The listing builds one solid part. Answer for the finished solid, in the listing's coordinates (mm). A direction names the side the tool comes from. Give positions to 0.01 mm unless a question says otherwise; leave off trailing zeros. Loops run counter-clockwise (first coordinate to the right, second up) from the corner with the lowest first, then second, coordinate; pieces in that order, holes last.
Item 1: Section A-A, the plane y = -91 is taken. Give the vertices of the cut face in (x, z), and give its area (3 significant figures).
Item 2: Section B-B, the plane x = 27 is taken. Give the vertices of the cut face in (y, z), and give its area (3 significant figures).
Item 3: Section C-C, the plane z = 31 is taken. Give the vertices of the cut face in (x, y).
Item 4: Each of these flat-tipped pins is pushed along its axis until it touches: pin 1 Ø20 at (x, z) = (15, 16) entering from +Y; pin 2 Ø2.5 at (y, z) = (-1.5, 0.5) entering from +X; pin 3 Ø1.5 at (x, y) = (33.5, -141) entering from +Z. Where does it stop, or does it pass through?
Item 5: A tool of negligible diameter and unlimited length cuts with its end or side. For faces 1 (the face through (35.5, -99, 0)), 2 (the face through (0, -32, 1.5)), 3 (the face through (-45.5, -95, 1)), from which of +Z, -Z, +X, -X, +Y, -Y can it reach the whole face along a straight path? Write none if from no direction.
Item 6: Consider line 1 along Y through (x, z) = (-38.5, 16); line 2 along Z through (x, y) = (-40, -45.5). Determine where each line is inside the solid, lowest interval first.
Autodesk Inventor part; units mm, degrees
ref_plane "YZ Plane" through (0, 0, 0) normal (1, 0, 0) x (0, 1, 0)
ref_plane "XZ Plane" through (0, 0, 0) normal (0, 1, 0) x (-1, 0, 0)
ref_plane "XY Plane" through (0, 0, 0) normal (0, 0, 1) x (1, 0, 0)
sketch "Skizze1" plane through (0, 0, 0) normal (0, 0, 1) x (1, 0, 0)
  line L0 (-45.5, 35.5) -> (45.5, 35.5)
  line L1 (45.5, 35.5) -> (45.5, -35.5)
  line L2 (45.5, -35.5) -> (-45.5, -35.5)
  line L3 (-45.5, -35.5) -> (-45.5, 35.5)
  line L4 (-45.5, 35.5) -> (45.5, -35.5) construction
  line L5 (45.5, 35.5) -> (-45.5, -35.5) construction
  line L6 (-34.8, 25.15) -> (45.5, 25.15)
  line L7 (-34.8, -25.15) -> (45.5, -25.15)
  line L8 (0, 0) -> (46.8412, 0)
  line L9 (-34.8, 25.15) -> (-34.8, -25.15)
  line L10 (-31.8, 25.15) -> (-40.5715, 16.3785)
  line L11 (-31.8, 25.15) -> (-19.3953, 25.15) construction
  point P0 (-34.8, 22.15)
  dimension "d0" = 91
  dimension "d1" = 71
  dimension "d4" = 80.3
  dimension "d5" = 50.3
  dimension "d23" = 135
  dimension "d24" = 3
extrude "Extrusion1" add sketch "Skizze1" along normal mid plane 3 contours L0 L1 L6 L9 L7 L2 L3 | L10 L9 L6
sketch "Skizze3" plane through (45.5, 25.15, 1.5) normal (1, 0, 0) x (0, 0, -1)
  line L0 (3, 0) -> (0, 0)
  line L1 (0, 0) -> (1.5, -0.866)
  line L2 (0, 0) -> (1.5, 0) construction
  line L3 (3, -50.3) -> (0, -50.3)
  line L4 (1.5, 0) -> (1.5, -50.3)
  line L5 (1.5, -0.866) -> (3, 0)
  line L6 (1.5, -25.15) -> (8.6012, -25.15)
  line L7 (0, -50.3) -> (1.5, -49.434)
  line L8 (1.5, -49.434) -> (3, -50.3)
  dimension "d7" = 30
extrude "Extrusion2" add sketch "Skizze3" against normal up to surface (80.3 mm away)
sketch "Skizze4" plane through (-45.5, -35.5, 1.5) normal (0, -1, 0) x (1, 0, 0)
  line L0 (0, 0) -> (91, 0)
  line L1 (91, -3) -> (0, -3)
  line L2 (0, 0) -> (10, 0)
  line L3 (10, 0) -> (10, -3)
  line L4 (10, -3) -> (0, -3)
  line L5 (0, -3) -> (0, 0)
  line L6 (91, -3) -> (91, 0)
  line L7 (91, -3) -> (81, -3)
  line L8 (81, -3) -> (81, 0)
  line L9 (81, 0) -> (91, 0)
  line L10 (91, 0) -> (91, -3)
  point P0 (45.5, -1.5)
  point P1 (81, 0)
  point P2 (81, -3)
  dimension "d10" = 10
  dimension "d11" = 10
extrude "Extrusion3" add sketch "Skizze4" along normal blind 130 contours L0 L3 L1 L5 | L0 L6 L1 L8
chamfer "Fase1" distance 3 angle 45 2 edges at (-35.5, -35.5, 0) (35.5, -35.5, 0)
sketch "Skizze6" plane through (0, 0, -1.5) normal (0, 0, -1) x (-1, 0, 0)
  line L0 (45.5, 35.5) -> (45.5, -165.5)
  line L1 (-45.5, -25.15) -> (-45.5, -165.5)
  line L2 (45.5, -165.5) -> (-45.5, -165.5)
  line L3 (-45.5, -165.5) -> (-45.5, -160.5)
  line L4 (-45.5, -160.5) -> (45.5, -160.5)
  line L5 (45.5, -160.5) -> (45.5, -165.5)
  point P0 (0, 0)
  dimension "d20" = 5
extrude "Extrusion5" add sketch "Skizze6" against normal blind 40
chamfer "Fase2" distance 3 angle 45 2 edges at (-40.5, -160.5, 1.5) (40.5, -160.5, 1.5)
equation "\"d11\" = d10"
properties part number "PiScanMiniDomeHolder"
Worked answers:
1. outline: (-45.5, -1.5) - (-35.5, -1.5) - (-35.5, 1.5) - (-45.5, 1.5) - close; (35.5, -1.5) - (45.5, -1.5) - (45.5, 1.5) - (35.5, 1.5) - close
1. area: 60.0 mm2
2. outline: (-165.5, -1.5) - (-160.5, -1.5) - (-160.5, 38.5) - (-165.5, 38.5) - close; (-35.5, -1.5) - (-25.15, -1.5) - (-24.28, 0) - (-25.15, 1.5) - (-35.5, 1.5) - close; (24.28, 0) - (25.15, -1.5) - (35.5, -1.5) - (35.5, 1.5) - (25.15, 1.5) - close
2. area: 265 mm2
3. outline: (-45.5, -165.5) - (45.5, -165.5) - (45.5, -160.5) - (-45.5, -160.5) - close
4. pin 1: stops at y = -160.5
4. pin 2: stops at x = -34.8
4. pin 3: passes through
5. face 1: +Z, -Z
5. face 2: +Z, +X, -X, +Y
5. face 3: +Z, -Z, -X, +Y, -Y
6. line 1: y = -165.5 to -160.5
6. line 2: z = -1.5 to 1.5
